Can you work these out from the model? Positions are in its coordinate system, mm. Coordinates: 2 decimals unless noted, no trailing zeros. Loops run counter-clockwise (first coordinate to the right, second up) from the corner with the lowest first, then second, coordinate; pieces in that order, holes last.
```python
from build123d import *

# Parameters (mm, degrees)
F0_R     = 3
F1_DEPTH = 3
F2_SIZE  = 2


with BuildPart() as f1:
    # F0 (on Front) → F1 (new body)
    with BuildSketch(Plane.XZ):
        with BuildLine():
            ThreePointArc((5, 0), (15, -10), (25, 0))
            ThreePointArc((25, 0), (0, 25), (-25, 0))
            ThreePointArc((-25, 0), (-23.515691, -5.242423), (-19.5034, -8.928571))
            ThreePointArc((-19.5034, -8.928571), (-12.820251, -14.739516), (-9.717181, -23.034244))
            ThreePointArc((-9.717181, -23.034244), (-9.698411, -23.213333), (-9.681434, -23.392601))
            Line((-9.681434, -23.392601), (-5.97037, -60.595556))
            ThreePointArc((-5.97037, -60.595556), (-4.026578, -64.448221), (0, -66))
            Line((0, -66), (0, -60))
            Line((0, -60), (0, -5))
            ThreePointArc((0, -5), (-3.535534, 3.535534), (5, 0))
        make_face()
        with Locations((-15, 0)):
            Circle(F0_R, mode=Mode.SUBTRACT)
        with Locations((15, 0)):
            Circle(F0_R, mode=Mode.SUBTRACT)
    extrude(amount=F1_DEPTH)

    # F2
    f2_edges = [f1.edges().sort_by_distance(p)[0] for p in [
        (0, -3, -35.5),
    ]]
    chamfer(f2_edges, length=F2_SIZE)


solid = f1.part
```
Item 1: We'd pull the mould along X, two halves only. Please class faces 1 (the face through (-0.4, 0, -9.8)), 2 (the face through (-4, -1, 3)), 3 (the face through (15, -1, -10)), 4 (the face through (-7.852, -1.479, -41.734)): +X half, -X half, draft (parallel to the pull), parting line (faces both ways), or undercut.
Results are:
face 1: draft
face 2: undercut
face 3: undercut
face 4: -X half
Item 2: I'm going to push flat-ended pins straight in: P1, Ø1.1, axis at y = -0.5, z = -21.5, coming from the +X side; P2, Ø1, axis at y = -1.5, z = -23.5, coming from the -X side. Where does each tip first touch, or does it pass through?
Results are:
P1: stops at x = 0
P2: stops at x = -9.72
Item 3: Suppose I cut it at B-B, the plane x = 15. Please give me the cut outline in (y, z), plus the area to 3 significant figures.
Results are:
outline: (-3, -10) - (0, -10) - (0, -3) - (-3, -3) - close; (-3, 3) - (0, 3) - (0, 20) - (-3, 20) - close
area: 72.0 mm2
Item 4: I need wall thicknesses on line 1 along X through (y, z) = (-2.75, -7); line 2 along Z through (x, y) = (0, -1.9); line 3 along Z through (x, y) = (15, -0.15). Which ranges of each line are inside material? Lowest first, please.
Results are:
line 1: x = -22.14 to -1.75, 7.86 to 22.14
line 2: z = 5 to 25
line 3: z = -10 to -3, 3 to 20
Item 5: Suppose I cut it at A-A, the plane z = -8. Please give me the cut outline in (x, y), plus the area to 3 significant figures.
Results are:
outline: (-21, -3) - (-2, -3) - (0, -1) - (0, 0) - (-21, 0) - close; (9, -3) - (21, -3) - (21, 0) - (9, 0) - close
area: 97.0 mm2
Item 6: Suppose I cut it at C-C, the plane y = -1.55. Please give me the cut outline in (x, z).
Results are:
outline: (-25, 0) arc R10 ccw to (-19.5, -8.93) arc R18 cw to (-9.72, -23.03) arc R17.99 cw to (-9.68, -23.39) - (-5.97, -60.6) arc R6 ccw to (-0.55, -65.97) - (-0.55, -4.97) arc R5 cw (long way) to (5, 0) arc R10 ccw to (25, 0) arc R25 ccw to start; hole circle Ø6 at (-15, 0); hole circle Ø6 at (15, 0)
Item 7: Suppose I cut it at D-D, the plane x = -1. Please give me the cut outline in (y, z).
Results are:
outline: (-3, 4.9) - (0, 4.9) - (0, 24.98) - (-3, 24.98) - close; (-2, -65.92) - (0, -65.92) - (0, -4.9) - (-2, -4.9) - close
